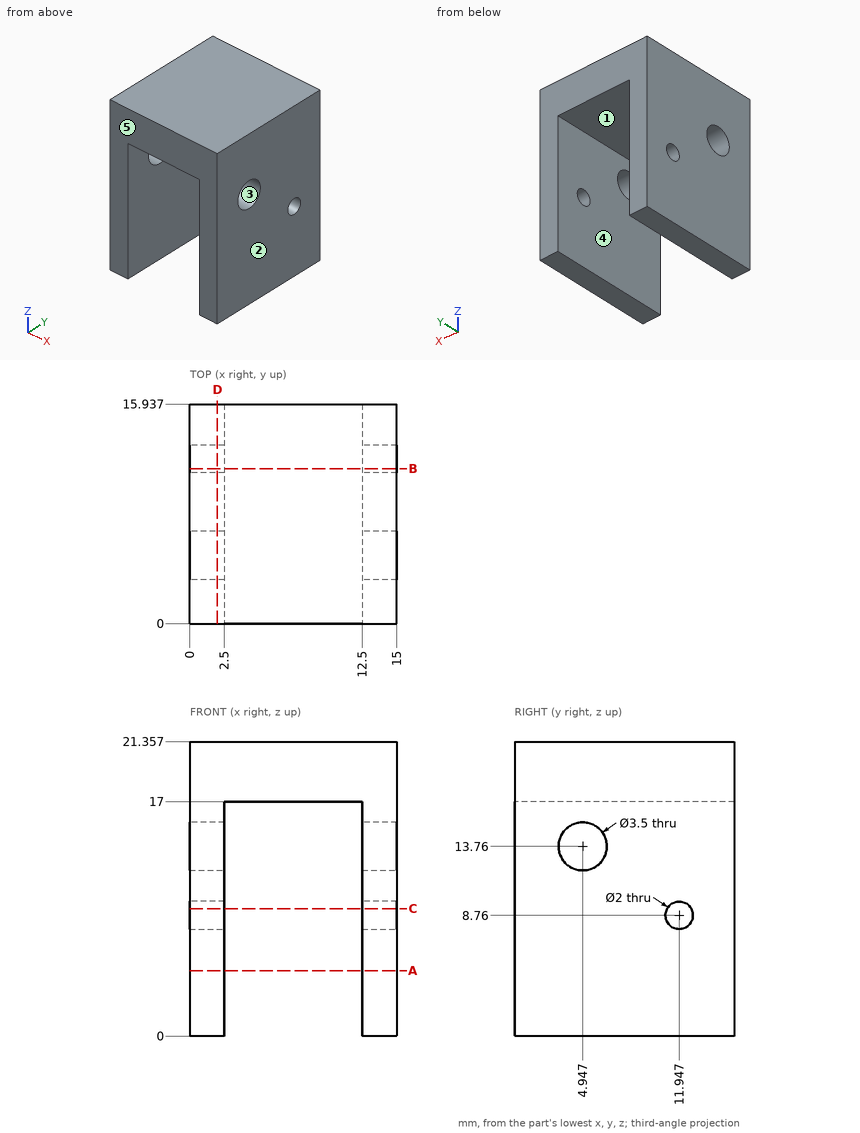
Job drawing, mm, ordinate dimensions from the low corner. One solid piece. A direction names the side the tool comes from. Coordinates: 2 decimals unless noted, no trailing zeros. Write each loop counter-clockwise with the first axis right and the second up, starting at its lowest first coordinate (ties: lowest second). Pieces come first, ordered by that corner, then holes. Notation, with made-up numbers: (8, -23.75) - (40, -23.75) arc R16 ccw to (40, -12.75) - close; hole circle Ø11 at (56.25, 84). An arc over 180 degrees is marked (long way). Use a Markdown table: item, result. Add a question column.
Item 1: Band-saw the part on A-A, the plane z = 4.75. Give the cut face in (x, y).
Item 2: Band-saw the part on C-C, the plane z = 9.25. Give the cut face in (x, y) (1 decimal).
Item 3: Band-saw the part on B-B, the plane y = 11.25. Give the cut face in (x, z), and give its area (3 significant figures).
Item 4: 3-axis set-ups, long thin cutter, end or side, ignore diameter. For the marked faces 4 and 5: which of +Z, -Z, +X, -X, +Y, -Y reach the whole face in a straight line?
Item 5: Band-saw the part on D-D, the plane x = 2. Give the cut face in (y, z).
Item 6: Drill centre lines: L1, parallel to X at y = 11.25, z = 12.5; L2, parallel to Z at x = 10, y = 13.25; L3, parallel to Y at x = 2, z = 9 (1 decimal). Where is each one in solid material? Low to high. Write a range as from..to.
Item 7: Flat gauge pins, fed straight in: pin 1 (5.5 mm diameter, centred on y = 4.95, z = 13.76, fed in from -X); pin 2 (5 mm diameter, centred on x = 7.5, y = 7, fed in from -Z). Where does each tip first touch, or does it go through?
Item 8: Mould opens along Z. For the marked faces 1, 2 and 3 say: pulls with the +Z half, pulls with the -Z half, needs draft (parallel to the pull), parting line crosses it, or undercut.
Numbers:
| question | item | result |
|---|---|---|
| 1 | outline | (0, 0) - (2.5, 0) - (2.5, 15.94) - (0, 15.94) - close; (12.5, 0) - (15, 0) - (15, 15.94) - (12.5, 15.94) - close |
| 2 | outline | (0, 0) - (2.5, 0) - (2.5, 11.1) - (0, 11.1) - close; (0, 12.8) - (2.5, 12.8) - (2.5, 15.9) - (0, 15.9) - close; (12.5, 0) - (15, 0) - (15, 11.1) - (12.5, 11.1) - close; (12.5, 12.8) - (15, 12.8) - (15, 15.9) - (12.5, 15.9) - close |
| 3 | outline | (0, 0) - (2.5, 0) - (2.5, 8.04) - (0, 8.04) - close; (0, 9.48) - (2.5, 9.48) - (2.5, 17) - (12.5, 17) - (12.5, 9.48) - (15, 9.48) - (15, 21.36) - (0, 21.36) - close; (12.5, 0) - (15, 0) - (15, 8.04) - (12.5, 8.04) - close |
| 3 | area | 143 mm2 |
| 4 | face 4 | -Z, +Y, -Y |
| 4 | face 5 | +Z, -Z, +X, -X, -Y |
| 5 | outline | (0, 0) - (15.94, 0) - (15.94, 21.36) - (0, 21.36) - close; hole circle Ø3.5 at (4.95, 13.76); hole circle Ø2 at (11.95, 8.76) |
| 6 | L1 | 0..2.5, 12.5..15 |
| 6 | L2 | 17..21.36 |
| 6 | L3 | 0..11, 12.9..15.9 |
| 7 | pin 1 | x = 0 |
| 7 | pin 2 | z = 17 |
| 8 | face 1 | pulls with the -Z half |
| 8 | face 2 | needs draft |
| 8 | face 3 | undercut |
